Part model, mm, in its own coordinate system. Round coordinates to 2 decimals unless told otherwise and drop trailing zeros. Loops run counter-clockwise (first coordinate to the right, second up) from the corner with the lowest first, then second, coordinate; pieces in that order, holes last.
from build123d import *

# Parameters (mm, degrees)
F1_W     = 70.58
F1_H     = 35.38
F2_DEPTH = 3.175
F0_R     = 1.09
F3_DEPTH = 3.176
F4_R     = 2


# Not quite as in the source:
# - a length typed as a fraction of an inch, garbled in the dataset ("3 / 203.2 mm" for 3/8 in), is restored


with BuildPart() as f2:
    # F1 (on Top) → F2 (new body)
    with BuildSketch(Plane.XY):
        Rectangle(F1_W, F1_H)
    extrude(amount=F2_DEPTH)

    # F0 (on Top) → F3 (cut, through all)
    with BuildSketch(Plane.XY):
        with Locations((-3, 14.6)):
            Circle(F0_R)
        with Locations((-3, -14.6)):
            Circle(F0_R)
        with Locations((-32.2, -14.6)):
            Circle(F0_R)
        with Locations((32.2, 14.6)):
            Circle(F0_R)
        with Locations((32.2, -14.6)):
            Circle(F0_R)
        with Locations((3, -14.6)):
            Circle(F0_R)
        with Locations((-32.2, 14.6)):
            Circle(F0_R)
        with Locations((3, 14.6)):
            Circle(F0_R)
    extrude(amount=F3_DEPTH, mode=Mode.SUBTRACT)

    # F4
    f4_edges = [f2.edges().sort_by_distance(p)[0] for p in [
        (-35.29, -17.69, 1.5875),
        (-35.29, 17.69, 1.5875),
        (35.29, 17.69, 1.5875),
        (35.29, -17.69, 1.5875),
    ]]
    fillet(f4_edges, radius=F4_R)


solid = f2.part
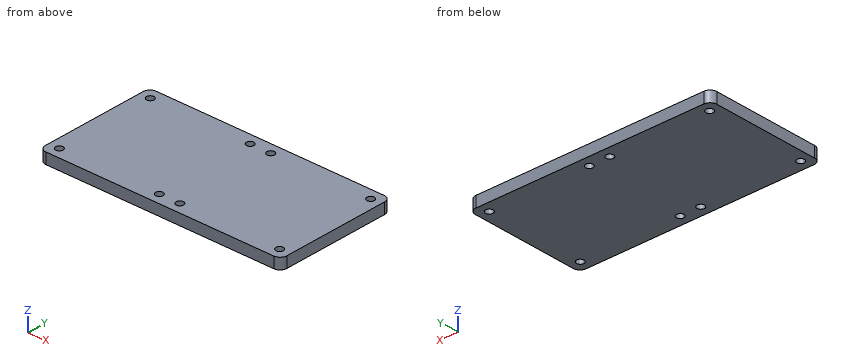
1) Slice it at A-A, the plane x = 32.2. Give the cut face in (y, z) (3 decimals), then the cut area to 3 significant figures.
Values:
outline: (-17.69, 0) - (-15.69, 0) - (-15.69, 3.175) - (-17.69, 3.175) - close; (-13.51, 0) - (13.51, 0) - (13.51, 3.175) - (-13.51, 3.175) - close; (15.69, 0) - (17.69, 0) - (17.69, 3.175) - (15.69, 3.175) - close
area: 98.5 mm2
2) Wall check: line 1 along X through (y, z) = (-14.5, 0.5); line 2 along Y through (x, z) = (-3, 2.4); line 3 along Y through (x, z) = (31.5, 1.8). Give the ranges that are in metal, low to high.
Values:
line 1: x = -35.29 to -33.29, -31.11 to -4.09, -1.91 to 1.91, 4.09 to 31.11, 33.29 to 35.29
line 2: y = -17.69 to -15.69, -13.51 to 13.51, 15.69 to 17.69
line 3: y = -17.69 to -15.44, -13.76 to 13.76, 15.44 to 17.69
3) Slice it at B-B, the plane y = -14.6. Give the cut face in (x, z) (3 decimals), then the cut area to 3 significant figures.
Values:
outline: (-35.29, 0) - (-33.29, 0) - (-33.29, 3.175) - (-35.29, 3.175) - close; (-31.11, 0) - (-4.09, 0) - (-4.09, 3.175) - (-31.11, 3.175) - close; (-1.91, 0) - (1.91, 0) - (1.91, 3.175) - (-1.91, 3.175) - close; (4.09, 0) - (31.11, 0) - (31.11, 3.175) - (4.09, 3.175) - close; (33.29, 0) - (35.29, 0) - (35.29, 3.175) - (33.29, 3.175) - close
area: 196 mm2
